Job drawing, mm, ordinate dimensions from the low corner. One solid piece. Give positions to 0.01 mm unless a question says otherwise; leave off trailing zeros. Order: outer loops, then holes, each group sorted by start corner. A loop starts at its lowest first (then second) coordinate and runs counter-clockwise, first axis right, second up.
Item 1: Band-saw the part on A-A on y = 1.75. Give the cut face in (x, z), plus the area to 3 significant figures.
Item 2: Two-plate mould, pull along X, no slides. Class the marked faces 1, 2 and 3: released by +X, released by -X, zero draft, split by the parting line, or undercut.
Item 3: Band-saw the part on D-D on x = 1.5. Give the cut face in (y, z), plus the area to 3 significant figures.
Item 4: Flat gauge pins, fed straight in: P1, Ø1.5, axis at x = 3, z = 1.5, coming from the +Y side; P2, Ø1, axis at x = 8, z = 0.5, coming from the +Y side (1 decimal). Where does each tip first touch, or does it go through?
Item 5: Wall check: L1, parallel to X at y = 6.25, z = 2.6 (1 decimal); L2, parallel to Y at x = 4.75, z = 1.9; L3, parallel to X at y = 3.25, z = 1.05. Give the ranges that are in metal, low to high.
Item 6: Band-saw the part on B-B on x = 4. Give the cut face in (y, z) (1 decimal).
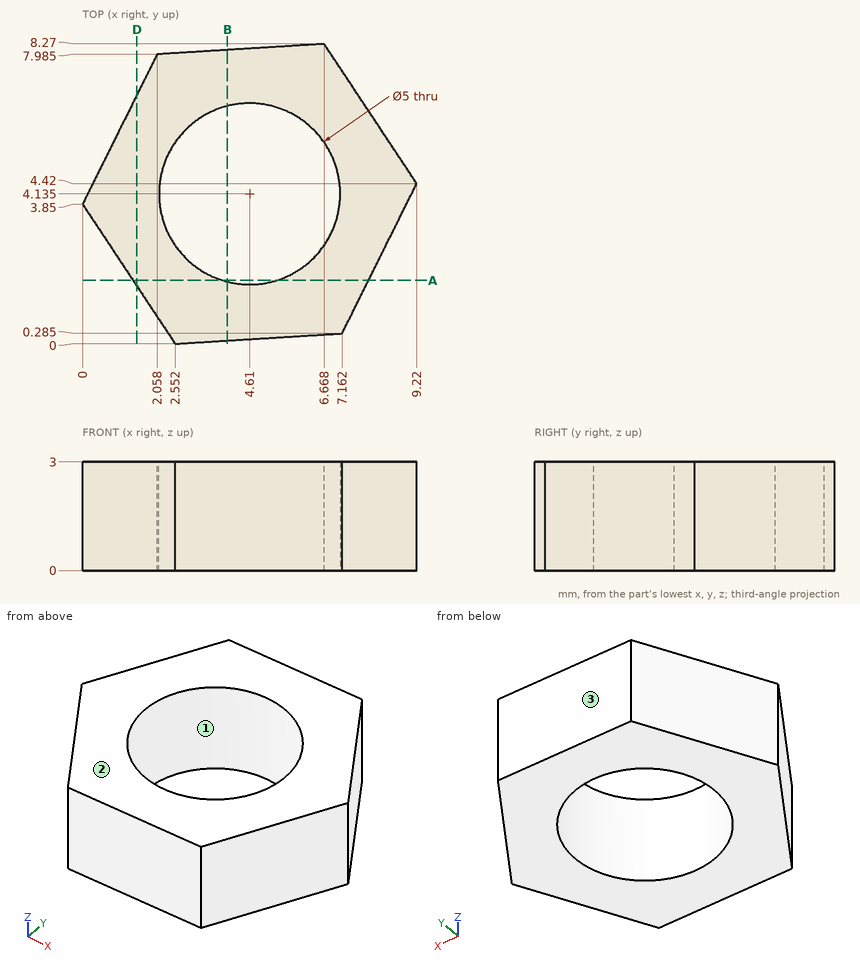
The answers:
1. outline: (1.39, 0) - (3.86, 0) - (3.86, 3) - (1.39, 3) - close; (5.36, 0) - (7.89, 0) - (7.89, 3) - (5.36, 3) - close
1. area: 15.0 mm2
2. face 1: undercut
2. face 2: zero draft
2. face 3: released by -X
3. outline: (1.59, 0) - (6.86, 0) - (6.86, 3) - (1.59, 3) - close
3. area: 15.8 mm2
4. P1: stops at y = 8.09
4. P2: stops at y = 7
5. L1: x = 1.2 to 3.3, 5.9 to 8
5. L2: y = 0.14 to 1.64, 6.63 to 8.15
5. L3: x = 0.4 to 2.27, 6.95 to 8.64
6. outline: (0.1, 0) - (1.7, 0) - (1.7, 3) - (0.1, 3) - close; (6.6, 0) - (8.1, 0) - (8.1, 3) - (6.6, 3) - close
